Here's the drawing with two shaded views (mm, measured from the low corner). I have some questions. Round coordinates to 2 decimals unless told otherwise and drop trailing zeros. Loops run counter-clockwise (first coordinate to the right, second up) from the corner with the lowest first, then second, coordinate; pieces in that order, holes last. Notation, with made-up numbers: (70.5, 76.25) -> (94.5, 76.25) arc R27 ccw to (94.5, 105.25) -> close; hole circle Ø5 at (-33, -22.5). An arc over 180 degrees is marked (long way). One line per item, written item: value. Start each with the question number.
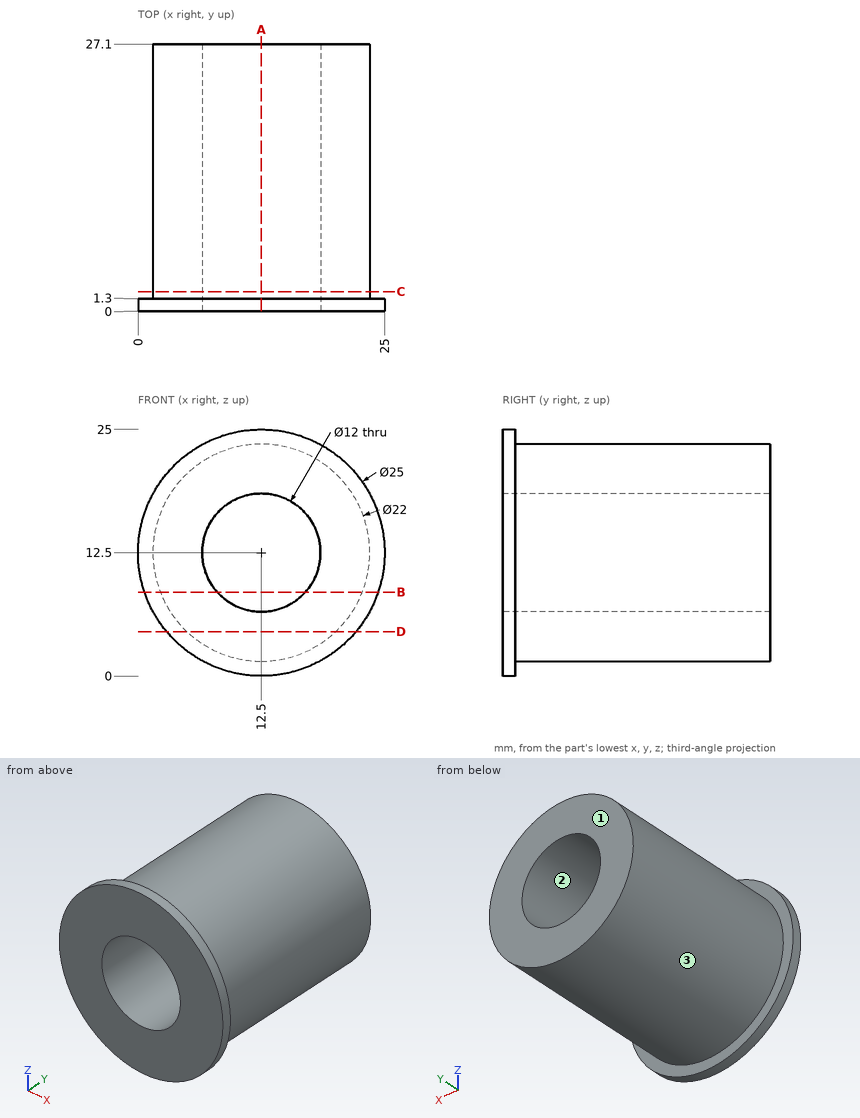
Q1. I want a section at D-D on z = 4.5. Please give me the cut outline in (x, y).
Q2. If I drill on line 1 along X through (y, z) = (16.75, 12.5); line 2 along Z through (x, y) = (16.25, 12); line 3 along Z through (x, y) = (15.75, 10.5), over which ranges is the centre line in solid material (lowest first)?
Q3. If we mould it in two halves opening along X, with no side actions, what happens to the marked faces 1, 2 and 3? For each: released by +X, released by -X, zero draft, split by the parting line, or undercut.
Q4. Will these pins go through, and if not, where does the flat tip stop? P1, Ø1, axis at x = 15.5, y = 13.5, coming from the -Z side; P2, Ø2, axis at y = 3.5, z = 22.5, coming from the -X side; P3, Ø8, axis at x = 6.5, y = 9.5, coming from the -Z side.
Q5. I want a section at B-B on z = 8.5. Please give me the cut outline in (x, y).
Q6. I want a section at C-C on y = 2. Please give me the cut outline in (x, z).
Q7. I want a section at A-A on x = 12.5. Please give me the cut outline in (y, z), plus the area to 3 significant figures.
Answers below:
1. outline: (2.9, 0) -> (22.1, 0) -> (22.1, 1.3) -> (20.05, 1.3) -> (20.05, 27.1) -> (4.95, 27.1) -> (4.95, 1.3) -> (2.9, 1.3) -> close
2. line 1: x = 1.5 to 6.5, 18.5 to 23.5
2. line 2: z = 2.16 to 7.82, 17.18 to 22.84
2. line 3: z = 1.99 to 7.46, 17.54 to 23.01
3. face 1: zero draft
3. face 2: undercut
3. face 3: split by the parting line
4. P1: stops at z = 1.79
4. P2: stops at x = 6.18
4. P3: stops at z = 1.68
5. outline: (0.66, 0) -> (8.03, 0) -> (8.03, 27.1) -> (2.25, 27.1) -> (2.25, 1.3) -> (0.66, 1.3) -> close; (16.97, 0) -> (24.34, 0) -> (24.34, 1.3) -> (22.75, 1.3) -> (22.75, 27.1) -> (16.97, 27.1) -> close
6. outline: circle Ø22 at (12.5, 12.5); hole circle Ø12 at (12.5, 12.5)
7. outline: (0, 0) -> (1.3, 0) -> (1.3, 1.5) -> (27.1, 1.5) -> (27.1, 6.5) -> (0, 6.5) -> close; (0, 18.5) -> (27.1, 18.5) -> (27.1, 23.5) -> (1.3, 23.5) -> (1.3, 25) -> (0, 25) -> close
7. area: 275 mm^2
